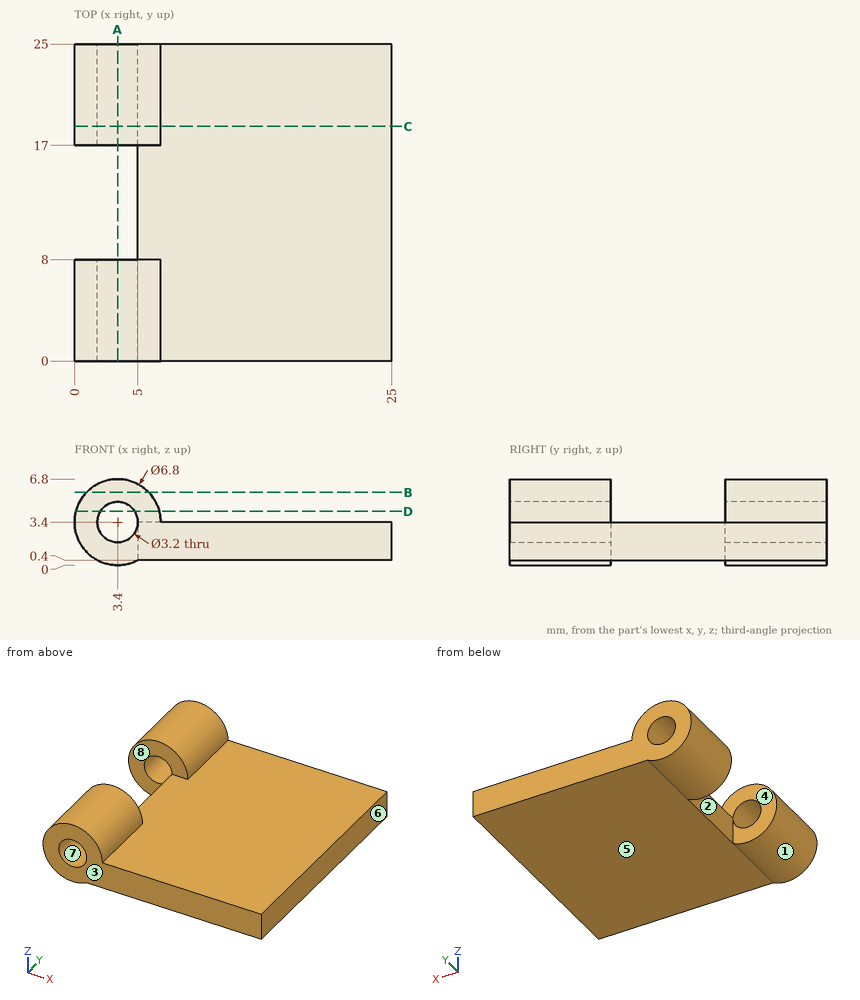
Input: dimensioned drawing with shaded views. Units: mm. Origin: part minimum x, y, z. A direction names the side the tool comes from. Give positions to 0.01 mm unless a question says otherwise; leave off trailing zeros. Order: outer loops, then holes, each group sorted by start corner. A loop starts at its lowest first (then second) coordinate and runs counter-clockwise, first axis right, second up.
(1) Section query D-D (z = 4.25). Return the cut outline in (x, y), plus the area to 3 significant figures.
(2) Section query C-C (y = 18.5). Return the cut outline in (x, z).
(3) Contact query for flat-ended pins moving along their axis: P1, Ø12, axis at x = 18, y = 12, coming from the -Z side; P2, Ø0.9, axis at y = 10.5, z = 1.5, coming from the -X side; P3, Ø2, axis at x = 3, z = 3.5, coming from the +Y side; P4, Ø12, axis at x = 21, y = 12.5, coming from the +Z side. Output: stop coordinate, or through.
(4) Section query B-B (z = 5.75). Return the cut outline in (x, y).
(5) Section query A-A (x = 3.4). Return the cut outline in (y, z), plus the area to 3 significant figures.
(6) Material intervals for line 1 along X through (y, z) = (2.25, 3.25); line 2 along Y through (x, z) = (1.5, 5); line 3 along Z through (x, y) = (11, 1.75), sorted ascending.
(7) Pull-direction query (X, two-part tool) for the marked faces 6, 7 and 8; classes: +X half, -X half, draft (parallel to the pull), parting line (faces both ways), or undercut.
(8) Access query for the marked faces 1, 2, 3, 4 and 5. Directions: +Z, -Z, +X, -X, +Y, -Y. A direction counts if a zero-diameter tool reaches every point of the face in a straight line with its end or side. Return the directions, or none.
Outcome:
1. outline: (0.11, 0) - (2.04, 0) - (2.04, 8) - (0.11, 8) - close; (0.11, 17) - (2.04, 17) - (2.04, 25) - (0.11, 25) - close; (4.76, 0) - (6.69, 0) - (6.69, 8) - (4.76, 8) - close; (4.76, 17) - (6.69, 17) - (6.69, 25) - (4.76, 25) - close
1. area: 62.0 mm2
2. outline: (5, 0.4) - (25, 0.4) - (25, 3.4) - (6.8, 3.4) arc R3.4 ccw (long way) to start; hole circle Ø3.2 at (3.4, 3.4)
3. P1: stops at z = 0.4
3. P2: stops at x = 5
3. P3: passes through
3. P4: stops at z = 3.4
4. outline: (0.94, 0) - (5.86, 0) - (5.86, 8) - (0.94, 8) - close; (0.94, 17) - (5.86, 17) - (5.86, 25) - (0.94, 25) - close
5. outline: (0, 0) - (8, 0) - (8, 1.8) - (0, 1.8) - close; (0, 5) - (8, 5) - (8, 6.8) - (0, 6.8) - close; (17, 0) - (25, 0) - (25, 1.8) - (17, 1.8) - close; (17, 5) - (25, 5) - (25, 6.8) - (17, 6.8) - close
5. area: 57.6 mm2
6. line 1: x = 0 to 1.81, 4.99 to 25
6. line 2: y = 0 to 8, 17 to 25
6. line 3: z = 0.4 to 3.4
7. face 6: +X half
7. face 7: undercut
7. face 8: draft
8. face 1: +Y, -Y
8. face 2: +Z, -Z, -X
8. face 3: +Z, -Z, +X, -X, -Y
8. face 4: +Z, -X
8. face 5: -Z, +X, +Y, -Y
